Model file for the job. Use its own axes, mm. A direction names the side the tool comes from. Coordinates: 2 decimals unless noted, no trailing zeros. Order: outer loops, then holes, each group sorted by start corner. A loop starts at its lowest first (then second) coordinate and runs counter-clockwise, first axis right, second up. Notation, with made-up numbers: (-4.75, 69.25) - (11.25, 69.25) arc R34 ccw to (11.25, 100.25) - close; hole circle Ø10 at (80.5, 11). An arc over 180 degrees is marked (long way). Put each result on its own line as item: value. Start each with the question number.
Autodesk Inventor part; units mm, degrees
ref_plane "YZ Plane" through (0, 0, 0) normal (1, 0, 0) x (0, 1, 0)
ref_plane "XZ Plane" through (0, 0, 0) normal (0, 1, 0) x (-1, 0, 0)
ref_plane "XY Plane" through (0, 0, 0) normal (0, 0, 1) x (1, 0, 0)
sketch "Sketch1" plane through (0, 0, 0) normal (0, 0, 1) x (1, 0, 0)
  line L0 (0, 0) -> (12, 0)
  line L1 (12, 0) -> (12, 12)
  line L2 (12, 12) -> (0, 12)
  line L3 (0, 12) -> (0, 0)
  line L4 (12, 0) -> (0, 0)
  line L5 (0, 0) -> (0, -12)
  line L6 (0, -12) -> (12, -12)
  line L7 (12, -12) -> (12, 0)
  line L8 (12, 0) -> (24, 0)
  line L9 (24, 0) -> (24, -12)
  line L10 (24, -12) -> (12, -12)
  line L11 (12, -12) -> (12, 0)
  line L12 (0, -12) -> (-12, -12)
  line L13 (-12, -12) -> (-12, 0)
  line L14 (-12, 0) -> (0, 0)
  line L15 (0, 0) -> (0, -12)
  line L16 (0, -12) -> (12, -12)
  line L17 (12, -12) -> (12, -24)
  line L18 (12, -24) -> (0, -24)
  line L19 (0, -24) -> (0, -12)
  dimension "d0" = 12
  dimension "d1" = 12
  dimension "d2" = 12
  dimension "d3" = 12
  dimension "d4" = 12
  dimension "d5" = 12
  dimension "d6" = 12
  dimension "d7" = 12
  dimension "d8" = 12
  dimension "d9" = 12
extrude "Extrusion1" add sketch "Sketch1" along normal blind 3
sketch "Sketch2" plane through (0, 0, 3) normal (0, 0, 1) x (1, 0, 0)
  line L0 (-12, 0) -> (-12, -12)
  line L1 (-12, -12) -> (-12, -6)
  line L2 (-12, -6) -> (0, -6)
  line L3 (-12, -12) -> (0, -12)
  line L4 (0, -6) -> (0, -12)
  line L5 (0, -12) -> (-12, -12)
  line L6 (12, -24) -> (12, -12)
  line L7 (12, -12) -> (12, -6)
  line L8 (12, -6) -> (24, -6)
  line L9 (24, -12) -> (24, 0)
  line L10 (12, -12) -> (24, -12)
  line L11 (24, -6) -> (24, -12)
  line L12 (24, -12) -> (12, -12)
  line L13 (0, 0) -> (0, -6)
  line L14 (12, 0) -> (12, 12)
  line L15 (0, 0) -> (12, 0)
  line L16 (12, 0) -> (12, -6)
  line L17 (12, -12) -> (0, -12)
  line L18 (0, 12) -> (0, 0)
  line L19 (0, 0) -> (0, 12)
  line L20 (0, 12) -> (6, 12)
  line L21 (12, 12) -> (0, 12)
  line L22 (6, 12) -> (6, 0)
  line L23 (6, 0) -> (0, 0)
  line L24 (0, -12) -> (0, -24)
  line L25 (0, -12) -> (0, -24)
  line L26 (0, -24) -> (6, -24)
  line L27 (0, -24) -> (12, -24)
  line L28 (6, -24) -> (6, -12)
  line L29 (6, -12) -> (0, -12)
  dimension "d12" = 6
  dimension "d13" = 12
extrude "Extrusion2" add sketch "Sketch2" along normal blind 9 contours L2 L4 L3 L0 | L13 L15 L16 L7 L17 L4 | L17 L28 L26 L24 | L18 L20 L22 L15 | L7 L8 L9 L10
sketch "Sketch3" plane through (0, 0, 12) normal (0, 0, 1) x (1, 0, 0)
  line L0 (0, -6) -> (12, -6)
  line L1 (12, -12) -> (6, -12)
  line L2 (12, -6) -> (12, -12)
  line L3 (0, -12) -> (0, -24)
  line L4 (12, -12) -> (0, -12)
  line L5 (0, -12) -> (0, -6)
  point P0 (0, 0)
extrude "Extrusion3" add sketch "Sketch3" along normal blind 9
sketch "Sketch4" plane through (6, -12, 3) normal (0, -1, 0) x (1, 0, 0)
  point P0 (-6, -3)
sketch "Sketch5" plane through (-12, -6, 3) normal (0, 1, 0) x (1, 0, 0)
  circle A0 centre (6, -4.5) radius 1.725
  line L0 (0, 0) -> (0, -9)
  line L1 (12, -9) -> (0, -9)
  circle A1 centre (18, -13.5) radius 1.725
  line L2 (24, -18) -> (12, -18)
  line L3 (24, -9) -> (24, -18)
  circle A2 centre (30, -4.5) radius 1.725
  line L4 (36, 0) -> (36, -9)
  line L5 (36, -9) -> (24, -9)
  point P0 (12, 3)
  dimension "d19" = 3.45
  dimension "d20" = 6
  dimension "d21" = 4.5
  dimension "d22" = 3.45
  dimension "d23" = 4.5
  dimension "d24" = 6
  dimension "d25" = 3.45
  dimension "d26" = 6
  dimension "d27" = 4.5
extrude "Extrusion4" cut sketch "Sketch5" against normal blind 3
sketch "Sketch6" plane through (6, -12, 3) normal (0, -1, 0) x (1, 0, 0)
  circle A0 centre (-12, 4.5) radius 1.725
  line L0 (-10.3546, 7.35) -> (-8.7091, 4.5)
  line L1 (-8.7091, 4.5) -> (-10.3546, 1.65)
  line L2 (-10.3546, 1.65) -> (-13.6454, 1.65)
  line L3 (-13.6454, 1.65) -> (-15.2909, 4.5)
  line L4 (-15.2909, 4.5) -> (-13.6454, 7.35)
  line L5 (-13.6454, 7.35) -> (-10.3546, 7.35)
  circle A1 centre (12, 4.5) radius 1.725
  line L6 (13.6454, 7.35) -> (15.2909, 4.5)
  line L7 (15.2909, 4.5) -> (13.6454, 1.65)
  line L8 (13.6454, 1.65) -> (10.3546, 1.65)
  line L9 (10.3546, 1.65) -> (8.7091, 4.5)
  line L10 (8.7091, 4.5) -> (10.3546, 7.35)
  line L11 (10.3546, 7.35) -> (13.6454, 7.35)
  circle A2 centre (0, 13.5) radius 1.725
  line L12 (1.6454, 16.35) -> (3.2909, 13.5)
  line L13 (3.2909, 13.5) -> (1.6454, 10.65)
  line L14 (1.6454, 10.65) -> (-1.6454, 10.65)
  line L15 (-1.6454, 10.65) -> (-3.2909, 13.5)
  line L16 (-3.2909, 13.5) -> (-1.6454, 16.35)
  line L17 (-1.6454, 16.35) -> (1.6454, 16.35)
  point P0 (-6, -3)
  dimension "d30" = 2.85
  dimension "d31" = 2.85
  dimension "d32" = 2.85
extrude "Extrusion5" cut sketch "Sketch6" against normal blind 3 contours A0 | L0 L1 L2 L3 L4 L5 | A1 | L6 L7 L8 L9 L10 L11 | A2 | L12 L13 L14 L15 L16 L17
sketch "Sketch7" plane through (6, 0, 3) normal (1, 0, 0) x (0, 0, -1)
  circle A0 centre (-4.5, 6) radius 1.725
  circle A1 centre (-4.5, -18) radius 1.725
  line L0 (-9, 0) -> (-9, 12)
  line L1 (-9, -24) -> (-9, -12)
  line L2 (0, -24) -> (-9, -24)
  line L3 (0, 12) -> (-9, 12)
  point P0 (3, 0)
  dimension "d35" = 3.45
  dimension "d36" = 3.45
  dimension "d37" = 4.5
  dimension "d38" = 4.5
  dimension "d39" = 6
  dimension "d40" = 6
extrude "Extrusion6" cut sketch "Sketch7" against normal blind 3
sketch "Sketch8" plane through (0, -6, 3) normal (-1, 0, 0) x (0, 0, 1)
  circle A0 centre (4.5, 12) radius 1.725
  line L0 (1.65, 13.6454) -> (4.5, 15.2909)
  line L1 (4.5, 15.2909) -> (7.35, 13.6454)
  line L2 (7.35, 13.6454) -> (7.35, 10.3546)
  line L3 (7.35, 10.3546) -> (4.5, 8.7091)
  line L4 (4.5, 8.7091) -> (1.65, 10.3546)
  line L5 (1.65, 10.3546) -> (1.65, 13.6454)
  circle A1 centre (4.5, -12) radius 1.725
  line L6 (1.65, -10.3546) -> (4.5, -8.7091)
  line L7 (4.5, -8.7091) -> (7.35, -10.3546)
  line L8 (7.35, -10.3546) -> (7.35, -13.6454)
  line L9 (7.35, -13.6454) -> (4.5, -15.2909)
  line L10 (4.5, -15.2909) -> (1.65, -13.6454)
  line L11 (1.65, -13.6454) -> (1.65, -10.3546)
  point P0 (-3, 6)
  dimension "d43" = 2.85
  dimension "d44" = 2.85
extrude "Extrusion7" cut sketch "Sketch8" against normal blind 3 contours A0 | L0 L1 L2 L3 L4 L5 | A1 | L6 L7 L8 L9 L10 L11
sketch "Sketch9" plane through (0, 0, 12) normal (0, 0, 1) x (1, 0, 0)
  line L0 (1.5, -10.5) -> (0, -12)
  line L1 (12, -12) -> (6, -12)
  line L2 (0, -12) -> (12, -12)
  line L3 (12, -24) -> (12, -12)
  line L4 (12, -12) -> (12, -24)
  line L5 (1.5, -24) -> (0, -24)
  line L6 (12, -24) -> (0, -24)
  line L7 (0, -24) -> (0, -12)
  line L8 (0, -12) -> (-12, -12)
  point P0 (0, 0)
extrude "Extrusion8" cut sketch "Sketch9" against normal blind 12
fillet "Fillet2" radius 1.5 3 edges at (6, -12, 0) (0, 6, 0) (12, 6, 0)
fillet "Fillet3" radius 1.5 2 edges at (0.75, 0, 0) (11.25, 0, 0)
properties part number "threewayVer1"
Item 1: Slice it at C-C, the plane x = -6. Give the cut face in (y, z) (3 decimals).
Item 2: Slice it at A-A, the plane x = 2. Give the cut face in (y, z), plus the area to 3 significant figures.
Item 3: Slice it at D-D, the plane y = 2.25. Give the cut face in (x, z), plus the area to 3 significant figures.
Item 4: Flat gauge pins, fed straight in: pin 1 Ø5 at (y, z) = (-9, 15) entering from -X; pin 2 Ø3 at (x, y) = (-3, -2) entering from +Z; pin 3 Ø4.5 at (x, z) = (18, 7.5) entering from -Y; pin 4 Ø8 at (y, z) = (8.5, 19) entering from -X. Where does each tip first touch, or does it go through?
Item 5: 3-axis set-ups, long thin cutter, end or side, ignore diameter. For faces 4 (the face through (6, -11, 19.35)), 5 (the face through (6, -6, 14)), 6 (the face through (18, -9, 12)): which of +Z, -Z, +X, -X, +Y, -Y reach the whole face in a straight line?
Item 6: Wall check: line 1 along X through (y, z) = (-7.25, 7.5) (3 decimals); line 2 along Y through (x, z) = (4.55, 7.5) (3 decimals); line 3 along Z through (x, y) = (18, -8) (3 decimals). Give the ranges that are in metal, low to high.
Item 7: Slice it at B-B, the plane y = 6. Give the cut face in (x, z) (3 decimals).
Item 8: Pull direction X, two halves, no side cores. Call faces 1 (the face through (-8.46, -10.52, 6.06)), 2 (the face through (24, -9, 5)), 3 (the face through (1.48, 8.46, 6.06)): pulls with the +X half, pulls with the -X half, needs draft (parallel to the pull), parting line crosses it, or undercut.
Here are the results:
1. outline: (-12, 1.5) arc R1.5 ccw to (-10.5, 0) - (-1.5, 0) arc R1.5 ccw to (0, 1.5) - (0, 3) - (-6, 3) - (-6, 5.775) - (-9, 5.775) - (-9, 4.65) - (-12, 4.65) - close; (-12, 10.35) - (-9, 10.35) - (-9, 9.225) - (-6, 9.225) - (-6, 12) - (-12, 12) - close
2. outline: (-12, 1.5) arc R1.5 ccw to (-10.5, 0) - (12, 0) - (12, 12) - (-6, 12) - (-6, 21) - (-12, 21) - close; hole (2.71, 7.5) - (4.35, 4.65) - (7.65, 4.65) - (9.29, 7.5) - (7.65, 10.35) - (4.35, 10.35) - close
2. area: 313 mm^2
3. outline: (0, 1.5) arc R1.5 ccw to (1.5, 0) - (10.5, 0) arc R1.5 ccw to (12, 1.5) - (12, 3) - (6, 3) - (6, 12) - (0, 12) - close
3. area: 89.0 mm^2
4. pin 1: stops at x = 0
4. pin 2: stops at z = 3
4. pin 3: stops at y = -9
4. pin 4: passes through
5. face 4: -Y
5. face 5: +Z, +X, -X, +Y
5. face 6: +Z, +X, +Y, -Y
6. line 1: x = -12 to -7.725, -4.275 to 16.275, 19.725 to 24
6. line 2: y = -12 to 4.275, 7.725 to 12
6. line 3: z = 0 to 5.775, 9.225 to 12
7. outline: (0, 1.5) arc R1.5 ccw to (1.5, 0) - (10.5, 0) arc R1.5 ccw to (12, 1.5) - (12, 3) - (6, 3) - (6, 5.775) - (3, 5.775) - (3, 4.65) - (0, 4.65) - close; (0, 10.35) - (3, 10.35) - (3, 9.225) - (6, 9.225) - (6, 12) - (0, 12) - close
8. face 1: undercut
8. face 2: pulls with the +X half
8. face 3: needs draft
